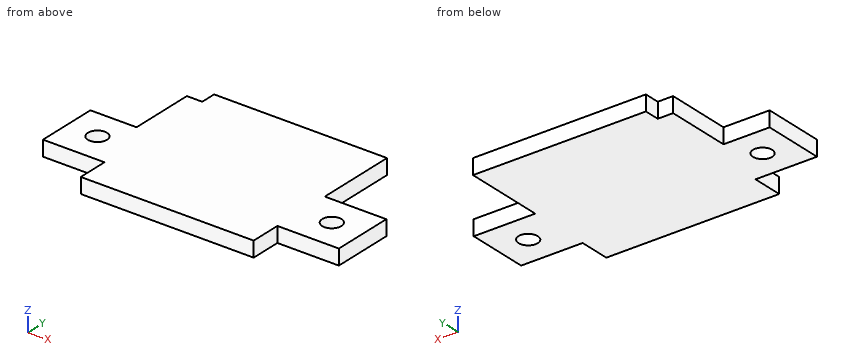
Solid Edge part; units mm, degrees
sketch "Sketch1" plane through (0, 0, 0) normal (0, 0, 1) x (1, 0, 0)
  line L0 (-11.25, -11.25) -> (11.25, -11.25)
  line L1 (11.25, -11.25) -> (11.25, 11.25)
  line L2 (11.25, 11.25) -> (-11.25, 11.25)
  line L3 (-11.25, 11.25) -> (-11.25, -11.25)
  dimension "D1" = 11.25
  dimension "D2" = 11.25
extrude "Protrusion1" add sketch "Sketch1" along normal blind 2
sketch "Sketch2" plane through (0, 0, 2) normal (0, 0, 1) x (1, 0, 0)
  line L0 (11.25, -7.25) -> (19.25, -7.25)
  line L1 (19.25, -7.25) -> (19.25, 0.75)
  line L2 (19.25, 0.75) -> (11.25, 0.75)
  line L3 (11.25, 0.75) -> (11.25, -7.25)
  dimension "D1" = 19.25
extrude "Protrusion2" add sketch "Sketch2" against normal up to vertex (2 mm away)
sketch "Sketch3" plane through (4, 0, 2) normal (0, 0, 1) x (1, 0, 0)
  line L0 (-15.25, -7.25) -> (-23.25, -7.25)
  line L1 (-23.25, -7.25) -> (-23.25, 0.75)
  line L2 (-23.25, 0.75) -> (-15.25, 0.75)
  line L3 (-15.25, 0.75) -> (-15.25, -7.25)
extrude "Extrusionsausprägung_3" add sketch "Sketch3" against normal blind 2
sketch "Sketch4" plane through (0, 0, 2) normal (0, 0, 1) x (1, 0, 0)
  circle A0 centre (-15.25, -3.25) radius 1.25
  circle A1 centre (15.25, -3.25) radius 1.25
extrude "Cutout1" cut sketch "Sketch4" against normal through all
sketch "Sketch5" plane through (0, 0, 2) normal (0, 0, 1) x (1, 0, 0)
  line L0 (-11.25, 11.25) -> (-13.25, 11.25)
  line L1 (-13.25, 11.25) -> (-13.25, 0.75)
  line L2 (-13.25, 0.75) -> (-11.25, 0.75)
  line L3 (-11.25, 0.75) -> (-11.25, 11.25)
  dimension "D1" = 11.25
extrude "Protrusion3" add sketch "Sketch5" against normal up to vertex (2 mm away)
sketch "Sketch6" plane through (0, 0, 2) normal (0, 0, 1) x (1, 0, 0)
  line L0 (-13.25, 11.25) -> (-11.25, 11.25)
  line L1 (-11.25, 11.25) -> (-11.25, 9.25)
  line L2 (-11.25, 9.25) -> (-13.25, 9.25)
  line L3 (-13.25, 9.25) -> (-13.25, 11.25)
  dimension "D1" = 11.25
  dimension "D2" = 11.25
extrude "Cutout2" cut sketch "Sketch6" against normal through all
Build history of the part. All positions in model axes, mm. Round coordinates to 2 decimals unless told otherwise and drop trailing zeros. Write each loop counter-clockwise with the first axis right and the second up, starting at its lowest first coordinate (ties: lowest second). Pieces come first, ordered by that corner, then holes. Notation, with made-up numbers: M 11.5,51.5 L 37.5,51.5 A21 ccw 37.5,67.5 Z; hole C -40,86.5 d7. An arc over 180 degrees is marked long. Answer as a JSON object with one key per item and string values. Group by question number.
(1) Cut at D-D (x = 15.5). Give the cut face in (y, z).
(2) Drill centre lines: L1, parallel to Y at x = -15.25, z = 0.8; L2, parallel to X at y = -3.5, z = 0.4; L3, parallel to X at y = 7.5, z = 0.6. Where is each one in solid material? Low to high.
(3) Cut at A-A (y = -3.25). Give the cut face in (x, z), and give its area (3 significant figures).
(4) Flat gauge pins, fed straight in: pin 1 (0.6 mm diameter, centred on x = 14.5, z = 1, fed in from +Y); pin 2 (1 mm diameter, centred on y = -9.5, z = 1, fed in from +X); pin 3 (1 mm diameter, centred on x = -15, z = 1.5, fed in from -Y). Where does each tip first touch, or does it go through?
(5) Cut at C-C (z = 0.3). Give the cut face in (x, y).
(6) Cut at B-B (x = -15.25). Give the cut face in (y, z), and give its area (3 significant figures).
Responses:
{
 "1": {"outline": "M -7.25,0 L -4.47,0 L -4.47,2 L -7.25,2 Z; M -2.03,0 L 0.75,0 L 0.75,2 L -2.03,2 Z"},
 "2": {"L1": "y = -7.25 to -4.5, -2 to 0.75", "L2": "x = -19.25 to -16.47, -14.03 to 14.03, 16.47 to 19.25", "L3": "x = -13.25 to 11.25"},
 "3": {"outline": "M -19.25,0 L -16.5,0 L -16.5,2 L -19.25,2 Z; M -14,0 L 14,0 L 14,2 L -14,2 Z; M 16.5,0 L 19.25,0 L 19.25,2 L 16.5,2 Z", "area": "67.0 mm2"},
 "4": {"pin 1": "stops at y = 0.75", "pin 2": "stops at x = 11.25", "pin 3": "stops at y = -7.25"},
 "5": {"outline": "M -19.25,-7.25 L -11.25,-7.25 L -11.25,-11.25 L 11.25,-11.25 L 11.25,-7.25 L 19.25,-7.25 L 19.25,0.75 L 11.25,0.75 L 11.25,11.25 L -11.25,11.25 L -11.25,9.25 L -13.25,9.25 L -13.25,0.75 L -19.25,0.75 Z; hole C -15.25,-3.25 d2.5; hole C 15.25,-3.25 d2.5"},
 "6": {"outline": "M -7.25,0 L -4.5,0 L -4.5,2 L -7.25,2 Z; M -2,0 L 0.75,0 L 0.75,2 L -2,2 Z", "area": "11.0 mm2"}
}
